Geometry check sheet. Reference: drawing and pictorial views, mm from the part's lowest x, y, z. Give positions to 0.01 mm unless a question says otherwise; leave off trailing zeros. Order: outer loops, then holes, each group sorted by start corner. A loop starts at its lowest first (then second) coordinate and runs counter-clockwise, first axis right, second up. Notation, with made-up numbers: (66.5, 17.5) - (89.5, 17.5) arc R18 ccw to (89.5, 45.5) - close; hole circle Ø8 at (-16.75, 84). An arc over 180 degrees is marked (long way). Answer in a Markdown table with one row per item.
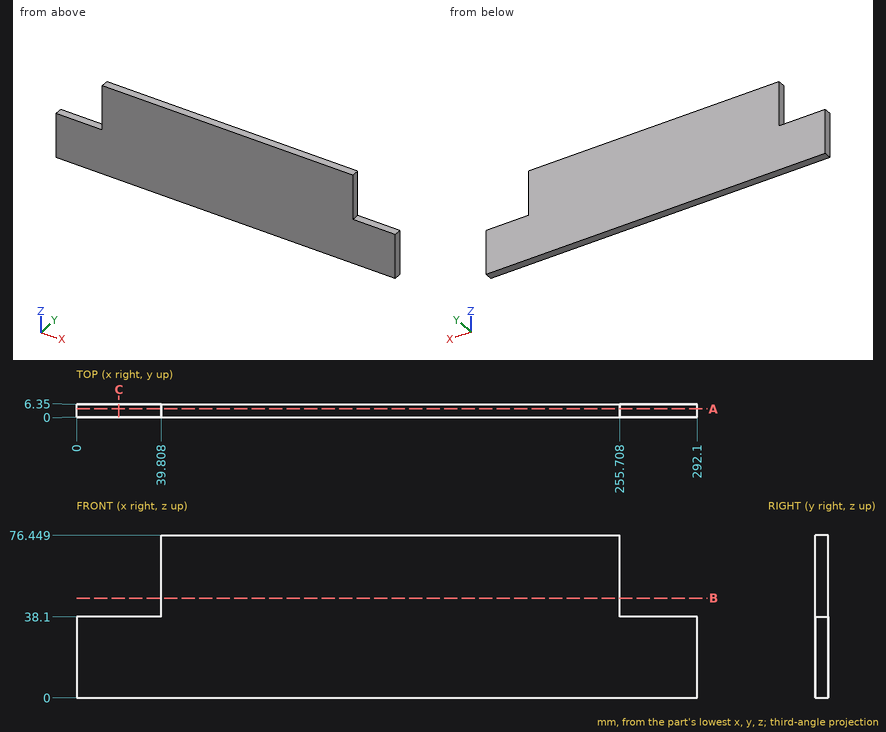
(1) Cross-section at B-B, the plane z = 47. Record the cut outline in (x, y), then the cut area to 3 significant figures.
Geometry says:
| item | result |
|---|---|
| outline | (39.81, 0) - (255.71, 0) - (255.71, 6.35) - (39.81, 6.35) - close |
| area | 1,370 mm² |
(2) Thickness scan on L1, parallel to X at y = 2.5, z = 49; L2, parallel to Z at x = 278, y = 4. Record the ranges inside material, lowest first.
Geometry says:
| item | result |
|---|---|
| L1 | 39.81 to 255.71 |
| L2 | 0 to 38.1 |
(3) Cross-section at C-C, the plane x = 20. Record the cut outline in (y, z), then the cut area to 3 significant figures.
Geometry says:
| item | result |
|---|---|
| outline | (0, 0) - (6.35, 0) - (6.35, 38.1) - (0, 38.1) - close |
| area | 242 mm² |
(4) Cross-section at A-A, the plane y = 4. Record the cut outline in (x, z).
Geometry says:
| item | result |
|---|---|
| outline | (0, 0) - (292.1, 0) - (292.1, 38.1) - (255.71, 38.1) - (255.71, 76.45) - (39.81, 76.45) - (39.81, 38.1) - (0, 38.1) - close |
(5) Gauge pin test, flat ends, axial feed: P1, Ø1.9, axis at x = 13.5, y = 4.5, coming from the +Z side; P2, Ø3, axis at y = 3.5, z = 51, coming from the +X side; P3, Ø1.9, axis at y = 2.5, z = 54.5, coming from the -X side. Record the tip position at first contact, or that the pin passes through.
Geometry says:
| item | result |
|---|---|
| P1 | z = 38.1 |
| P2 | x = 255.71 |
| P3 | x = 39.81 |
